Design review of the part built by this model. Coordinates are the model's own, in mm. A direction names the side the tool comes from. Give positions to 0.01 mm unless a question says otherwise; leave off trailing zeros. Order: outer loops, then holes, each group sorted by start corner. A loop starts at its lowest first (then second) coordinate and runs counter-clockwise, first axis right, second up. Notation, with made-up numbers: (-1, -27) -> (11, -27) arc R25 ccw to (11, 12) -> close; hole circle Ø3 at (-11, 24.25). An arc over 180 degrees is marked (long way). Return JSON: item names as keys, results as strings.
```python
from build123d import *

# Parameters (mm, degrees)
SKETCH_1_R          = 20
SKETCH_1_R_2        = 2.5
EXTRUDE_1_DEPTH     = 7
SKETCH_2_R          = 12
EXTRUDE_2_DEPTH     = 8
SKETCH_3_R          = 2.6
CUT_EXTRUDE_1_DEPTH = 7
SKETCH_4_R          = 3.1
CUT_EXTRUDE_2_DEPTH = 1
SKETCH_6_R          = 3.1
CUT_EXTRUDE_3_DEPTH = 1


with BuildPart() as part:
    # Эскиз1 → Бобышка-Вытянуть1 (new body)
    with BuildSketch(Plane.XY):
        Circle(SKETCH_1_R)
        with Locations((-10.5, 10.5)):
            Circle(SKETCH_1_R_2, mode=Mode.SUBTRACT)
        with Locations((10.5, 10.5)):
            Circle(SKETCH_1_R_2, mode=Mode.SUBTRACT)
        with Locations((10.5, -10.5)):
            Circle(SKETCH_1_R_2, mode=Mode.SUBTRACT)
        with Locations((-10.5, -10.5)):
            Circle(SKETCH_1_R_2, mode=Mode.SUBTRACT)
    extrude(amount=EXTRUDE_1_DEPTH)

    # Эскиз2 → Бобышка-Вытянуть2 (add)
    with BuildSketch(Plane.XY.offset(7)):
        Circle(SKETCH_2_R)
    extrude(amount=EXTRUDE_2_DEPTH)

    # Эскиз3 → Вырез-Вытянуть1 (cut)
    with BuildSketch(Plane.XY.offset(15)):
        with Locations((-8, 0)):
            Circle(SKETCH_3_R)
        with Locations((0, 8)):
            Circle(SKETCH_3_R)
        with Locations((8, 0)):
            Circle(SKETCH_3_R)
        with Locations((0, -8)):
            Circle(SKETCH_3_R)
    extrude(amount=-CUT_EXTRUDE_1_DEPTH, mode=Mode.SUBTRACT)

    # Эскиз4 → Вырез-Вытянуть2 (cut)
    with BuildSketch(Plane.XY.offset(15)):
        with Locations((-8, 0)):
            Circle(SKETCH_4_R)
        with Locations((0, 8)):
            Circle(SKETCH_4_R)
        with Locations((8, 0)):
            Circle(SKETCH_4_R)
        with Locations((0, -8)):
            Circle(SKETCH_4_R)
    extrude(amount=-CUT_EXTRUDE_2_DEPTH, mode=Mode.SUBTRACT)

    # Эскиз6 → Вырез-Вытянуть3 (cut)
    with BuildSketch(Plane.XY.offset(8)):
        with Locations((8, 0)):
            Circle(SKETCH_6_R)
        with Locations((0, 8)):
            Circle(SKETCH_6_R)
        with Locations((-8, 0)):
            Circle(SKETCH_6_R)
        with Locations((0, -8)):
            Circle(SKETCH_6_R)
    extrude(amount=-CUT_EXTRUDE_3_DEPTH, mode=Mode.SUBTRACT)


solid = part.part
```
Item 1: Machinability: for faces 1 (the face through (9.96, 8.06, 3.45)), 2 (the face through (-2, -10, 14)), 3 (the face through (-0.404, 11.074, 7.507)), which of the approach directions +Z, -Z, +X, -X, +Y, -Y give a long, thin tool a straight path to every point of the face, cutting with its end or side? Answer none if there is none.
Result set:
{"face 1": "+Z, -Z", "face 2": "+Z", "face 3": "none"}
Item 2: Add section D-D (y = -9.5). Give the boundary of the cut face in (x, z).
Result set:
{"outline": "(-17.6, 0) -> (-12.79, 0) -> (-12.79, 7) -> (-17.6, 7) -> close; (-8.21, 0) -> (8.21, 0) -> (8.21, 7) -> (7.33, 7) -> (7.33, 15) -> (2.71, 15) -> (2.71, 14) -> (2.12, 14) -> (2.12, 8) -> (2.71, 8) -> (2.71, 7) -> (-2.71, 7) -> (-2.71, 8) -> (-2.12, 8) -> (-2.12, 14) -> (-2.71, 14) -> (-2.71, 15) -> (-7.33, 15) -> (-7.33, 7) -> (-8.21, 7) -> close; (12.79, 0) -> (17.6, 0) -> (17.6, 7) -> (12.79, 7) -> close"}
Item 3: For pin 1 (3 mm diameter, centred on x = -8, y = 0, fed in from +Z); pin 2 (4 mm diameter, centred on x = -10.5, y = 10.5, fed in from -Z); pin 3 (4 mm diameter, centred on x = 1.5, z = 6.5, fed in from +Y); pin 4 (3 mm diameter, centred on x = 0, y = 9.5, fed in from +Z), all flat-tipped, find the tip position at first contact; note any pin that passes through.
Result set:
{"pin 1": "stops at z = 7", "pin 2": "passes through", "pin 3": "stops at y = 20", "pin 4": "stops at z = 14"}
Item 4: Add section A-A (z = 10.5). Give the boundary of the cut face in (x, y).
Result set:
{"outline": "circle Ø24 at (0, 0); hole circle Ø5.2 at (-8, 0); hole circle Ø5.2 at (0, -8); hole circle Ø5.2 at (0, 8); hole circle Ø5.2 at (8, 0)"}
Item 5: Mouldability with a two-part tool opening along X and no side actions: class faces 4 (the face through (8.6, -8.6, 7)), 5 (the face through (-4.336, -19.524, 3.451)), 6 (the face through (0, 8, 7)) as released by +X, released by -X, zero draft, split by the parting line, or undercut.
Result set:
{"face 4": "zero draft", "face 5": "split by the parting line", "face 6": "undercut"}
Item 6: Wall thickness on L1, parallel to Y at x = 0, z = 9.75; L2, parallel to Y at x = 0, z = 14.2; L3, parallel to X at y = 9.5, z = 2.5: over which ranges is each line inside the solid? List them lowest first. Write a range as [from, to].
Result set:
{"L1": "y = [-12, -10.6], [-5.4, 5.4], [10.6, 12]", "L2": "y = [-12, -11.1], [-4.9, 4.9], [11.1, 12]", "L3": "x = [-17.6, -12.79], [-8.21, 8.21], [12.79, 17.6]"}
